Part print with two shaded views. Sizes in mm from the minimum x, y, z corner. A direction names the side the tool comes from. Round coordinates to 2 decimals unless told otherwise and drop trailing zeros. Order: outer loops, then holes, each group sorted by start corner. A loop starts at its lowest first (then second) coordinate and runs counter-clockwise, first axis right, second up. Notation, with made-up numbers: M 84.5,79 L 100.5,79 A32 ccw 100.5,118 Z; hole C -16.5,34 d2. An arc over 180 degrees is marked long. One line per question, with ' | ' between items.
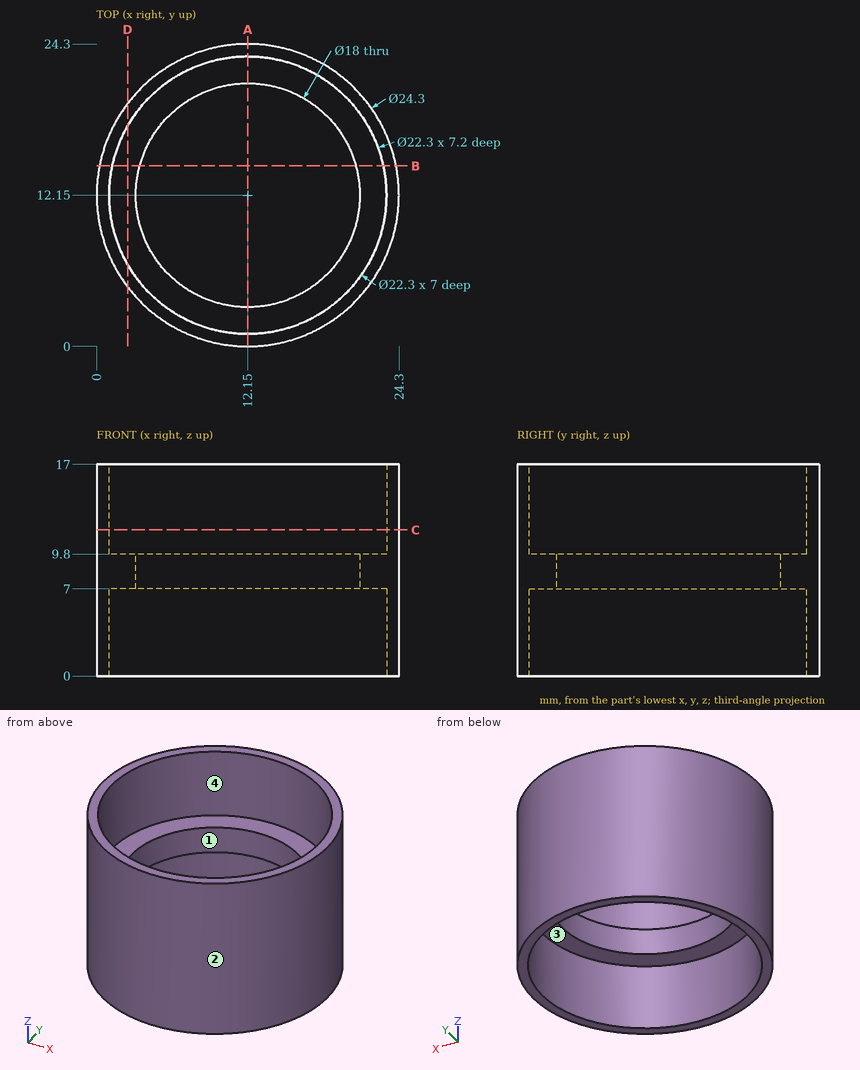
1) Probe line 1 (Y direction, x = 12.15, z = 8.4); line 2 (Y direction, x = 12.15, z = 15.75); line 3 (X direction, y = 13, z = 11.25). List the from-to ranges inside material, lowest first. Write a range as [from, to].
The answers:
line 1: y = [0, 3.15], [21.15, 24.3] | line 2: y = [0, 1], [23.3, 24.3] | line 3: x = [0.03, 1.03], [23.27, 24.27]
2) Saw through at A-A (x = 12.15). List the corners of the cut face in (y, z).
The answers:
outline: M 0,0 L 1,0 L 1,7 L 3.15,7 L 3.15,9.8 L 1,9.8 L 1,17 L 0,17 Z; M 21.15,7 L 23.3,7 L 23.3,0 L 24.3,0 L 24.3,17 L 23.3,17 L 23.3,9.8 L 21.15,9.8 Z
3) Saw through at B-B (y = 14.5). List the corners of the cut face in (x, z), plus the area to 3 significant figures.
The answers:
outline: M 0.23,0 L 1.25,0 L 1.25,7 L 3.46,7 L 3.46,9.8 L 1.25,9.8 L 1.25,17 L 0.23,17 Z; M 20.84,7 L 23.05,7 L 23.05,0 L 24.07,0 L 24.07,17 L 23.05,17 L 23.05,9.8 L 20.84,9.8 Z | area: 47.1 mm²
4) Which spindle directions (+Z, -Z, +X, -X, +Y, -Y) get a long thin tool onto all of the face, cutting with end or side? Do the marked faces 3 and 4. Say none if no direction does.
The answers:
face 3: -Z | face 4: +Z
5) Two-plate mould, pull along X, no slides. Class the marked faces 1 and 2: released by +X, released by -X, zero draft, split by the parting line, or undercut.
The answers:
face 1: undercut | face 2: split by the parting line
6) Saw through at D-D (x = 2.5). List the corners of the cut face in (y, z).
The answers:
outline: M 4.77,0 L 6.56,0 L 6.56,7 L 17.74,7 L 17.74,0 L 19.53,0 L 19.53,17 L 17.74,17 L 17.74,9.8 L 6.56,9.8 L 6.56,17 L 4.77,17 Z
7) Saw through at C-C (z = 11.75). List the corners of the cut face in (x, y).
The answers:
outline: C 12.15,12.15 d24.3; hole C 12.15,12.15 d22.3
8) Drop flat-ended pins along their axis: pin 1 (2 mm diameter, centred on x = 17, z = 4.5, fed in from -Y); pin 2 (3 mm diameter, centred on y = 8.5, z = 13, fed in from -X); pin 3 (5 mm diameter, centred on x = 15, z = 15.5, fed in from -Y); pin 4 (14.5 mm diameter, centred on x = 12.15, y = 12.15, fed in from -Z). Give the stop position or say it passes through.
The answers:
pin 1: stops at y = 0.63 | pin 2: stops at x = 0.19 | pin 3: stops at y = 0.01 | pin 4: passes through
